Read the model definition and answer for the solid it produces. Units are mm, in the model's axes. A direction names the side the tool comes from. Give positions to 0.01 mm unless a question says otherwise; leave off trailing zeros. Write each loop counter-clockwise with the first axis right and the second up, starting at its lowest first coordinate (ties: lowest second). Pieces come first, ordered by that corner, then holes.
```python
from build123d import *

# Parameters (mm, degrees)
F0_W     = 18
F0_H     = 48
F1_DEPTH = 2
F0_W_2   = 4
F0_H_2   = 0.775
F0_H_3   = 1.05
F2_DEPTH = 2.5
F0_H_4   = 0.45
F3_DEPTH = 4
F4_R     = 1


with BuildPart() as f1:
    # F0 (on Top) → F1 (new body)
    with BuildSketch(Plane.XY):
        with Locations((0, 16)):
            Rectangle(F0_W, F0_H)
        Polygon((2.04878, -3.225), (2.04878, -4), (-1.95122, -4), (-1.95122, -3.225), (-1.95122, -2.775), (-1.95122, -1.725), (-1.95122, -1.275), (-1.95122, -0.225), (-1.95122, 0), (-1.95122, 0.107463), (-1.95122, 0.225), (-1.95122, 1.275), (-1.95122, 1.725), (-1.95122, 2.775), (-1.95122, 3.225), (-1.95122, 4), (2.04878, 4), (2.04878, 3.225), (2.04878, 2.775), (2.04878, 1.725), (2.04878, 1.275), (2.04878, 0.225), (2.04878, -0.225), (2.04878, -1.275), (2.04878, -1.725), (2.04878, -2.775), align=None, mode=Mode.SUBTRACT)
    extrude(amount=F1_DEPTH)

    # F0 (on Top) → F2 (join)
    with BuildSketch(Plane.XY):
        with Locations((0.04878, -3.6125)):
            Rectangle(F0_W_2, F0_H_2)
        with Locations((0.04878, -2.25)):
            Rectangle(F0_W_2, F0_H_3)
        with Locations((0.04878, -0.75)):
            Rectangle(F0_W_2, F0_H_3)
        with Locations((0.04878, 0.75)):
            Rectangle(F0_W_2, F0_H_3)
        with Locations((0.04878, 2.25)):
            Rectangle(F0_W_2, F0_H_3)
        with Locations((0.04878, 3.6125)):
            Rectangle(F0_W_2, F0_H_2)
    extrude(amount=F2_DEPTH)

    # F0 (on Top) → F3 (join)
    with BuildSketch(Plane.XY):
        with Locations((0.04878, -3)):
            Rectangle(F0_W_2, F0_H_4)
        with Locations((0.04878, -1.5)):
            Rectangle(F0_W_2, F0_H_4)
        Polygon((-1.95122, -0.225), (2.04878, -0.225), (2.04878, 0.225), (-1.95122, 0.225), (-1.95122, 0.107463), (-1.95122, 0), align=None)
        with Locations((0.04878, 1.5)):
            Rectangle(F0_W_2, F0_H_4)
        with Locations((0.04878, 3)):
            Rectangle(F0_W_2, F0_H_4)
    extrude(amount=F3_DEPTH)

    # F4
    f4_edges = [f1.edges().sort_by_distance(p)[0] for p in [
        (9, 16, 0),
        (-9, 16, 0),
        (0, -8, 0),
        (-9, 40, 1),
        (9, -8, 1),
        (-9, -8, 1),
    ]]
    fillet(f4_edges, radius=F4_R)


solid = f1.part
```
Item 1: Determine the mould class of faces 6 (the flat face through (0, 2, 2.5)), 7 (the cylindrical face through (8.715, -7.699, 1.507)), 8 (the cylindrical face through (-8.699, 39.715, 1.236)) for opening direction Y: pulls with the +Y half, pulls with the -Y half, needs draft (parallel to the pull), parting line crosses it, or undercut.
Result set:
face 6: undercut
face 7: pulls with the -Y half
face 8: pulls with the +Y half
Item 2: Find the intervals of material crossed by line 1 along Z through (x, y) = (4.25, 17.5); line 2 along Z through (x, y) = (1.25, 1); line 3 along X through (y, z) = (-0.5, 2.4), in increasing order.
Result set:
line 1: z = 0 to 2
line 2: z = 0 to 2.5
line 3: x = -1.95 to 2.05
Item 3: Section C-C (y = 7.5) is taken. Write down the section's boundary in (x, z).
Result set:
outline: (-9, 1) arc R1 ccw to (-8, 0) - (8, 0) arc R1 ccw to (9, 1) - (9, 2) - (-9, 2) - close
Item 4: Section A-A (z = 3.3) is taken. Write down the section's boundary in (x, y) (3 decimals), and give its area (3 significant figures).
Result set:
outline: (-1.951, -3.225) - (2.049, -3.225) - (2.049, -2.775) - (-1.951, -2.775) - close; (-1.951, -1.725) - (2.049, -1.725) - (2.049, -1.275) - (-1.951, -1.275) - close; (-1.951, -0.225) - (2.049, -0.225) - (2.049, 0.225) - (-1.951, 0.225) - close; (-1.951, 1.275) - (2.049, 1.275) - (2.049, 1.725) - (-1.951, 1.725) - close; (-1.951, 2.775) - (2.049, 2.775) - (2.049, 3.225) - (-1.951, 3.225) - close
area: 9.00 mm2
Item 5: Section D-D (x = 3.5) is taken. Write down the section's boundary in (y, z).
Result set:
outline: (-8, 1) arc R1 ccw to (-7, 0) - (40, 0) - (40, 2) - (-8, 2) - close
Item 6: Each of these flat-tipped pins is pushed along its axis until it touches: pin 1 Ø1.6 at (x, z) = (0, 3.5) entering from -Y (3 decimals); pin 2 Ø0.8 at (x, z) = (-0.5, 3.5) entering from +Y (3 decimals); pin 3 Ø1.6 at (x, z) = (0.5, 3) entering from -Y. Where does it stop, or does it pass through?
Result set:
pin 1: stops at y = -3.225
pin 2: stops at y = 3.225
pin 3: stops at y = -4
Item 7: Which of the six approach directions +Z, -Z, +X, -X, +Y, -Y give full straight-line access (tool end or side, diameter ignored) to faces 1 (the flat face through (0, 3.225, 3)), 2 (the flat face through (0, -3.225, 3)), 3 (the flat face through (-1.951, 0, 3)), 4 (the flat face through (2.049, 0, 3)), 5 (the flat face through (0, -2.775, 3))?
Result set:
face 1: +Z, +X, -X, +Y
face 2: +Z, +X, -X, -Y
face 3: +Z, -X, +Y, -Y
face 4: +Z, +X, +Y, -Y
face 5: +Z, +X, -X
